```python
from build123d import *

# Parameters (mm, degrees)
EXTRUDE_THIN1_DEPTH = 635
FILLET1_R           = 1.27


with BuildPart() as part:
    # Sketch1 → Extrude-Thin1 (new body)
    with BuildSketch(Plane.XY):
        with BuildLine():
            Line((0, 0), (-5.55625, 0))
            Line((-5.55625, 0), (-5.55625, 3.175))
            ThreePointArc((-5.55625, 3.175), (-9.775089119, 5.089375145), (-11.1125, 9.525))
            Line((-11.1125, 9.525), (-14.2875, 9.525))
            Line((-14.2875, 9.525), (-14.2875, 42.247372018))
            ThreePointArc((-14.2875, 42.247372018), (-16.976339174, 47.831898282), (-23.01875, 49.2125))
            Line((-23.01875, 49.2125), (-23.01875, 66.675))
            Line((-23.01875, 66.675), (0, 66.675))
            Line((0, 66.675), (0, 65.405))
            Line((0, 65.405), (-21.74875, 65.405))
            Line((-21.74875, 65.405), (-21.74875, 50.655129317))
            ThreePointArc((-21.74875, 50.655129317), (-15.595162979, 48.308005429), (-13.0175, 42.247372018))
            Line((-13.0175, 42.247372018), (-13.0175, 10.795))
            Line((-13.0175, 10.795), (-9.395900253, 10.795))
            ThreePointArc((-9.395900253, 10.795), (-8.89341428, 6.012644953), (-4.28625, 4.635165643))
            Line((-4.28625, 4.635165643), (-4.28625, 1.27))
            Line((-4.28625, 1.27), (0, 1.27))
            Line((0, 1.27), (0, 0))
        make_face()
    extrude(amount=-EXTRUDE_THIN1_DEPTH)

    # Fillet1
    fillet1_edges = [part.edges().sort_by_distance(p)[0] for p in [
        (-9.395900253, 10.795, -317.5),
        (-4.28625, 4.635165643, -317.5),
        (-5.55625, 0, -317.5),
        (-14.2875, 9.525, -317.5),
        (-23.01875, 49.2125, -317.5),
        (-23.01875, 66.675, -317.5),
    ]]
    fillet(fillet1_edges, radius=FILLET1_R)


solid = part.part
```
Geometry check sheet. Reference: the model listing, model coordinates, mm. A direction names the side the tool comes from. Give positions to 0.01 mm unless a question says otherwise; leave off trailing zeros. Order: outer loops, then holes, each group sorted by start corner. A loop starts at its lowest first (then second) coordinate and runs counter-clockwise, first axis right, second up. Notation, with made-up numbers: (35, 56) - (53, 56) arc R33 cw to (53, 92) - close; hole circle Ø4 at (-22.5, 58.25). An arc over 180 degrees is marked (long way). Write item = value, one per line. Start each with the question number.
1) Section check A-A (y = 23). Enter the section's corners in (x, z), then the cut area to 3 significant figures.
2) Access from +Z, -Z, +X, -X, +Y, -Y to the whole of each face (thin tool, end or side, straight path). Record for faces 1 (the flat face through (-23.019, 58, -313)), 2 (the flat face through (-14.288, 26, -313)), 3 (the flat face through (-13.018, 27, -313)).
3) Section check B-B (z = -286). Enter the section's corners in (x, y) (1 decimal), then the cut area to 3 significant figures.
4) Scan lines: L1, parallel to Y at x = -20.5, z = -60 (3 decimals); L2, parallel to Y at x = -3.75, z = -433.5 (3 decimals); L3, parallel to X at y = 57.5, z = -263. Record each from-to range of solid material in increasing order.
5) Gauge pin test, flat ends, axial feed: pin 1 Ø6.5 at (x, z) = (-14, -383.5) entering from -Y; pin 2 Ø6 at (y, z) = (47.5, -388) entering from +X; pin 3 Ø25 at (y, z) = (26, -192) entering from +X. Record the tip position at first contact, or that the pin passes through.
6) Draft check along Y on faces 4 (the flat face through (-11, 66.675, -313)), 5 (the flat face through (-13.2, 40.9, -635)), 6 (the flat face through (-11, 65.405, -313)). Enter one of: released by +Y, released by -Y, zero draft, split by the parting line, or undercut.
Geometry check:
q1.outline = (-14.29, -635) - (-13.02, -635) - (-13.02, 0) - (-14.29, 0) - close
q1.area = 806 mm2
q2.face_1 = +Z, -Z, -X, +Y, -Y
q2.face_2 = +Z, -Z, -X, -Y
q2.face_3 = +Z, -Z, +X
q3.outline = (-23, 50.7) arc R1.3 ccw to (-21.7, 49.4) arc R7.1 cw to (-14.3, 42.2) - (-14.3, 10.8) arc R1.3 ccw to (-13, 9.5) - (-11.1, 9.5) arc R5.6 ccw to (-5.6, 3.2) - (-5.6, 1.3) arc R1.3 ccw to (-4.3, 0) - (0, 0) - (0, 1.3) - (-4.3, 1.3) - (-4.3, 3.2) arc R1.3 ccw to (-5.6, 4.4) arc R4.3 cw to (-9.9, 9.4) arc R1.3 ccw to (-11.1, 10.8) - (-13, 10.8) - (-13, 42.2) arc R8.4 ccw to (-21.7, 50.7) - (-21.7, 65.4) - (0, 65.4) - (0, 66.7) - (-21.7, 66.7) arc R1.3 ccw to (-23, 65.4) - close
q3.area = 131 mm2
q4.L1 = 49.33 to 50.609, 65.405 to 66.675
q4.L2 = 0 to 1.27, 65.405 to 66.675
q4.L3 = -23.02 to -21.75
q5.pin_1 = 6.67
q5.pin_2 = -13.32
q5.pin_3 = -13.02
q6.face_4 = released by +Y
q6.face_5 = zero draft
q6.face_6 = undercut
